Autodesk Inventor part; units mm, degrees
ref_plane "YZ Plane" through (0, 0, 0) normal (1, 0, 0) x (0, 1, 0)
ref_plane "XZ Plane" through (0, 0, 0) normal (0, 1, 0) x (-1, 0, 0)
ref_plane "XY Plane" through (0, 0, 0) normal (0, 0, 1) x (1, 0, 0)
sketch "Sketch1" plane through (0, 0, 0) normal (0, 1, 0) x (-1, 0, 0)
  line L0 (0, 0) -> (-22.86, 0)
  line L1 (-22.86, 0) -> (-22.86, -22.86)
  line L2 (-22.86, -22.86) -> (0, -22.86)
  line L3 (0, -22.86) -> (0, 0)
  line L4 (-22.86, -22.86) -> (-19.304, -22.86)
  line L5 (-19.304, -22.86) -> (-19.304, -19.304) construction
  line L6 (-19.304, -19.304) -> (-22.86, -19.304) construction
  line L7 (-22.86, -19.304) -> (-22.86, -22.86)
  line L8 (0, -22.86) -> (-3.556, -22.86)
  line L9 (-3.556, -22.86) -> (-3.556, -19.304) construction
  line L10 (-3.556, -19.304) -> (0, -19.304) construction
  line L11 (0, -19.304) -> (0, -22.86)
  line L12 (0, 0) -> (-3.556, 0)
  line L13 (-3.556, 0) -> (-3.556, -3.556) construction
  line L14 (-3.556, -3.556) -> (0, -3.556) construction
  line L15 (0, -3.556) -> (0, 0)
  line L16 (-22.86, 0) -> (-19.304, 0)
  line L17 (-19.304, 0) -> (-19.304, -3.556) construction
  line L18 (-19.304, -3.556) -> (-22.86, -3.556) construction
  line L19 (-22.86, -3.556) -> (-22.86, 0)
  circle A0 centre (-3.556, -19.304) radius 2.075
  circle A1 centre (-19.304, -19.304) radius 2.075
  circle A2 centre (-19.304, -3.556) radius 2.075
  circle A3 centre (-3.556, -3.556) radius 2.075
  line L20 (3.57, -26.43) -> (-26.43, -26.43)
  line L21 (-26.43, -26.43) -> (-26.43, 3.57)
  line L22 (-26.43, 3.57) -> (3.57, 3.57)
  line L23 (3.57, 3.57) -> (3.57, -26.43)
  line L24 (0, 0) -> (-6.5, 0)
  line L25 (-6.5, 0) -> (-6.5, -6.5)
  line L26 (-6.5, -6.5) -> (0, -6.5)
  line L27 (0, -6.5) -> (0, 0)
  line L28 (0, -22.86) -> (-6.5, -22.86)
  line L29 (-6.5, -22.86) -> (-6.5, -16.36)
  line L30 (-6.5, -16.36) -> (0, -16.36)
  line L31 (0, -16.36) -> (0, -22.86)
  line L32 (-22.86, -22.86) -> (-16.36, -22.86)
  line L33 (-16.36, -22.86) -> (-16.36, -16.36)
  line L34 (-16.36, -16.36) -> (-22.86, -16.36)
  line L35 (-22.86, -16.36) -> (-22.86, -22.86)
  line L36 (-22.86, 0) -> (-16.36, 0)
  line L37 (-16.36, 0) -> (-16.36, -6.5)
  line L38 (-16.36, -6.5) -> (-22.86, -6.5)
  line L39 (-22.86, -6.5) -> (-22.86, 0)
  line L40 (-26.43, 3.57) -> (-49.205, 3.57)
  line L41 (-49.205, 3.57) -> (-49.205, -26.43)
  line L42 (-49.205, -26.43) -> (-26.43, -26.43)
  line L43 (-26.43, -26.43) -> (-26.43, 3.57)
  circle A4 centre (-11.43, -11.43) radius 5
  line L44 (-9.3887, -15.2384) -> (-13.3887, -15.2384)
  line L45 (-13.3887, -15.2384) -> (-13.3887, -23.9816)
  line L46 (-13.3887, -23.9816) -> (-9.3887, -23.9816)
  line L47 (-9.3887, -15.2384) -> (-13.3887, -23.9816) construction
  line L48 (-13.3887, -15.2384) -> (-9.3887, -23.9816) construction
  line L49 (5.2257, -13.68) -> (-9.4126, -13.68)
  line L50 (-9.4126, -13.68) -> (-9.4126, -9.18)
  line L51 (-9.4126, -9.18) -> (5.2257, -9.18)
  line L52 (5.2257, -9.18) -> (5.2257, -13.68)
  line L53 (5.2257, -13.68) -> (-9.4126, -9.18) construction
  line L54 (-9.4126, -13.68) -> (5.2257, -9.18) construction
  point P0 (0, -16.36)
  point P1 (0, -6.5)
  point P2 (-11.3887, -19.61)
  point P3 (-2.0935, -11.43)
  point P4 (0, -9.18)
  point P5 (3.57, -9.18)
  point P6 (3.57, -13.68)
  point P7 (0, -13.68)
  dimension "d2" = 22.86
  dimension "d3" = 22.86
  dimension "d4" = 3.556
  dimension "d5" = 3.556
  dimension "d6" = 3.556
  dimension "d7" = 3.556
  dimension "d8" = 3.556
  dimension "d9" = 3.556
  dimension "d10" = 3.556
  dimension "d11" = 3.556
  dimension "d12" = 4.15
  dimension "d13" = 4.15
  dimension "d14" = 4.15
  dimension "d15" = 4.15
  dimension "d16" = 30
  dimension "d17" = 30
  dimension "d18" = 3.57
  dimension "d19" = 3.57
  dimension "d20" = 6.5
  dimension "d21" = 6.5
  dimension "d22" = 6.5
  dimension "d23" = 6.5
  dimension "d24" = 6.5
  dimension "d25" = 6.5
  dimension "d26" = 6.5
  dimension "d31" = 10
  dimension "d32" = 15
  dimension "d33" = 15
  dimension "d34" = 37.775
  dimension "d69" = 4
  dimension "d70" = 4.5
extrude "Extrusion1" add sketch "Sketch1" along normal blind 7 contours L3 L26 L25 L0 | L0 L1 L2 L3 L49 L23 L20 L21 L22 L51 | L37 L38 L1 L0 | L3 L2 L29 L30 | L34 L33 L2 L1 | L21 L42 L41 L40
fillet "Fillet1" radius 2 4 edges at (6.5, 3.5, -16.36) (16.36, 3.5, -16.36) (16.36, 3.5, -6.5) (6.5, 3.5, -6.5)
sketch "Sketch4" plane through (49.205, 0, 3.57) normal (1, 0, 0) x (0, 0, -1)
  line L0 (-10, 13.5061) -> (40, 13.5061)
  line L1 (40, 13.5061) -> (40, -6.4939)
  line L2 (40, -6.4939) -> (-10, -6.4939)
  line L3 (-10, -6.4939) -> (-10, 13.5061)
  line L4 (-10, 13.5061) -> (40, -6.4939) construction
  line L5 (40, 13.5061) -> (-10, -6.4939) construction
  line L6 (30, 0) -> (30, 7)
  line L7 (15, 3.5061) -> (35, 3.5061)
  circle A0 centre (35, 3.5061) radius 1.65
  circle A1 centre (-5, 3.5061) radius 1.65
  line L8 (-10, 0) -> (40, 0)
  line L9 (40, 0) -> (40, 13.5061)
  line L10 (40, 13.5061) -> (-10, 13.5061)
  line L11 (-10, 13.5061) -> (-10, 0)
  line L12 (-10, -6.4939) -> (0, -6.4939)
  line L13 (0, -6.4939) -> (0, 0)
  line L14 (0, 0) -> (-10, 0)
  line L15 (-10, 0) -> (-10, -6.4939)
  line L16 (40, -6.4939) -> (30, -6.4939)
  line L17 (30, -6.4939) -> (30, 0)
  line L18 (30, 0) -> (40, 0)
  line L19 (40, 0) -> (40, -6.4939)
  line L20 (40, 13.5061) -> (20, 13.5061)
  line L21 (20, 13.5061) -> (20, 6.753)
  line L22 (20, 6.753) -> (40, 6.753)
  line L23 (40, 6.753) -> (40, 13.5061)
  line L24 (0, 7) -> (30, 7)
  line L25 (-10, 13.5061) -> (10, 13.5061)
  line L26 (10, 13.5061) -> (10, 7)
  line L27 (10, 7) -> (-10, 7)
  line L28 (-10, 7) -> (-10, 13.5061)
  point P0 (3.57, 0)
  point P1 (40, -3.247)
  point P2 (-10, -3.247)
  point P3 (-10, 10.253)
  point P4 (10, 10.253)
  point P5 (40, 10.1296)
  point P6 (20, 13.5061)
  point P7 (10, 13.5061)
  point P8 (-10, 7)
  point P9 (40, 6.753)
  dimension "d46" = 50
  dimension "d47" = 20
  dimension "d48" = 15
  dimension "d49" = 10
  dimension "d56" = 20
  dimension "d57" = 20
  dimension "d58" = 3.3
  dimension "d59" = 3.3
  dimension "d66" = 10
  dimension "d67" = 20
  dimension "d68" = 20
extrude "Extrusion4" add sketch "Sketch4" against normal blind 5 contours L0 L21 L24 L26 | L27 L24 L21 L22 L6 L8 L3 | L8 L13 L2 L3 | L8 L17 L2 L13 | L1 L8 L6 L22 | L8 L1 L2 L17
fillet "Fillet2" radius 5 2 edges at (-3.57, 3.5, -26.43) (-3.57, 3.5, 3.57)
chamfer "Chamfer1" distance 10 angle 45 2 edges at (46.705, -6.4939, 13.57) (46.705, -6.4939, -36.43)
sketch "Sketch5" plane through (0, 7, 0) normal (0, 1, 0) x (1, 0, 0)
  line L0 (-8.8762, -11.5964) -> (30.2556, -11.5964)
  line L1 (30.2556, -11.5964) -> (30.2556, 37.6524)
  line L2 (30.2556, 37.6524) -> (-8.8762, 37.6524)
  line L3 (-8.8762, 37.6524) -> (-8.8762, -11.5964)
  point P0 (0, 0)
extrude "Extrusion5" cut sketch "Sketch5" against normal blind 4
properties part number "as5600mount"
Check sheet for the modelled part. Datum: model origin and axes. Units: mm. A direction names the side the tool comes from. Round coordinates to 2 decimals unless told otherwise and drop trailing zeros. Loops run counter-clockwise (first coordinate to the right, second up) from the corner with the lowest first, then second, coordinate; pieces in that order, holes last. Notation, with made-up numbers: M 47,18.25 L 59,18.25 A10 cw 59,35.25 Z; hole C 15,-7.75 d7. An arc over 180 degrees is marked long. One line per question, with ' | ' between items. Start each with the question number.
Item 1: Scan lines: probe 1 along X at (y, z) = (0.5, -7.5) (3 decimals); probe 2 along Y at (x, z) = (11, 1.5); probe 3 along Y at (x, z) = (31, -18). Record each from-to range of solid material in increasing order.
Item 2: Set-up check for faces 1 (the face through (-2, 1, -9.18)), 2 (the face through (5.9, 1.52, -16.93)), 3 (the face through (27.9, 2.7, 3.57)): record each of +Z, -Z, +X, -X, +Y, -Y from which the full face is reachable in a straight line by a thin tool's end or side.
Item 3: Section check A-A (x = 45.5). Record the boundary of the cut face in (y, z).
Item 4: Gauge pin test, flat ends, axial feed: pin 1 Ø6 at (x, z) = (20.5, -1) entering from +Y; pin 2 Ø3 at (y, z) = (-2, -11) entering from -X (3 decimals); pin 3 Ø4 at (x, y) = (38, 7) entering from -Z; pin 4 Ø3 at (y, z) = (3.51, 8.57) entering from -X. Record the tip position at first contact, or that the pin passes through.
Item 5: Section check B-B (z = 9). Record the boundary of the cut face in (x, y) (3 decimals), and give its area (3 significant figures).
Item 6: Release check for a two-part mould opening along X. For faces 4 (the face through (-3.57, 1, -5)), 5 (the face through (5.93, 1.52, -5.9)), 6 (the face through (47, 5, 13.57)), 7 (the face through (49.205, 1, -11)) record: released by +X, released by -X, zero draft, split by the parting line, or undercut.
Item 7: Section check D-D (x = 26). Record the boundary of the cut face in (y, z).
Item 8: Section check C-C (z = -13). Record the boundary of the cut face in (x, y) (3 decimals).
Worked out:
1) probe 1: -3.57 to 0, 22.86 to 49.205 | probe 2: 0 to 3 | probe 3: 0 to 7
2) face 1: -X, +Y, -Y | face 2: +Y, -Y | face 3: +Z, -X, +Y, -Y
3) outline: M -6.49,-26.43 L 3.51,-36.43 L 6.75,-36.43 L 6.75,-26.43 L 7,-26.43 L 7,-16.43 L 13.51,-16.43 L 13.51,-6.43 L 7,-6.43 L 7,13.57 L 3.51,13.57 L -6.49,3.57 Z; hole C 3.51,-31.43 d3.3; hole C 3.51,8.57 d3.3
4) pin 1: y = 3 | pin 2: x = 44.205 | pin 3: z = -26.43 | pin 4: through
5) outline: M 44.205,-1.064 L 49.205,-1.064 L 49.205,1.913 L 44.205,1.913 Z; M 44.205,5.099 L 49.205,5.099 L 49.205,7 L 44.205,7 Z | area: 24.4 mm^2
6) face 4: released by -X | face 5: undercut | face 6: zero draft | face 7: released by +X
7) outline: M 0,-26.43 L 3,-26.43 L 3,3.57 L 0,3.57 Z
8) outline: M 22.86,0 L 44.205,0 L 44.205,-6.494 L 49.205,-6.494 L 49.205,13.506 L 44.205,13.506 L 44.205,7 L 30.256,7 L 30.256,3 L 22.86,3 Z
